Work out the finished part from the listing and answer in its coordinate system (mm). Face numbers are marked on the shaded views. A direction names the side the tool comes from. Round coordinates to 2 decimals unless told otherwise and drop trailing zeros. Loops run counter-clockwise (first coordinate to the right, second up) from the corner with the lowest first, then second, coordinate; pieces in that order, holes last.
from build123d import *

# Parameters (mm, degrees)
BOSS_EXTRUDE1_DEPTH = 30
SKETCH2_W           = 10
SKETCH2_H           = 20
SKETCH2_R           = 2.25
BOSS_EXTRUDE2_DEPTH = 4
SKETCH3_W           = 20
SKETCH3_H           = 10
CUT_EXTRUDE1_DEPTH  = 5
FILLET1_R           = 4
CHAMFER1_SIZE       = 14
CHAMFER1_SIZE2      = 16.684550296


with BuildPart() as part:
    # Sketch1 → Boss-Extrude1 (new body)
    with BuildSketch(Plane(origin=(0, 0, 0), x_dir=(0, 0, -1), z_dir=(1, 0, 0))):
        Polygon((0, 20), (20, 40), (20, 20), (20, 0), (0, 0), align=None)
    extrude(amount=BOSS_EXTRUDE1_DEPTH)

    # Sketch2 → Boss-Extrude2 (add)
    with BuildSketch(Plane.XY):
        with Locations((-5, 10)):
            Rectangle(SKETCH2_W, SKETCH2_H)
        with Locations((-5, 10)):
            Circle(SKETCH2_R, mode=Mode.SUBTRACT)
        with Locations((35, 10)):
            Rectangle(SKETCH2_W, SKETCH2_H)
        with Locations((35, 10)):
            Circle(SKETCH2_R, mode=Mode.SUBTRACT)
    extrude(amount=-BOSS_EXTRUDE2_DEPTH)

    # Sketch3 → Cut-Extrude1 (cut)
    with BuildSketch(Plane(origin=(0, 10, 10), x_dir=(1, 0, 0), z_dir=(0, 0.707106781, 0.707106781))):
        with Locations((15, 26.142135624)):
            Rectangle(SKETCH3_W, SKETCH3_H)
    extrude(amount=-CUT_EXTRUDE1_DEPTH, mode=Mode.SUBTRACT)

    # Fillet1
    fillet1_edges = [part.edges().sort_by_distance(p)[0] for p in [
        (15, 40, -20),
    ]]
    fillet(fillet1_edges, radius=FILLET1_R)

    # Chamfer1
    chamfer1_edges = [part.edges().sort_by_distance(p)[0] for p in [
        (15, 0, -20),
    ]]
    chamfer1_side = [part.faces().sort_by_distance(p)[0] for p in [
        (15, 0, -9.058823529),
    ]]
    chamfer(chamfer1_edges, length=CHAMFER1_SIZE, length2=CHAMFER1_SIZE2, reference=chamfer1_side[0])


solid = part.part
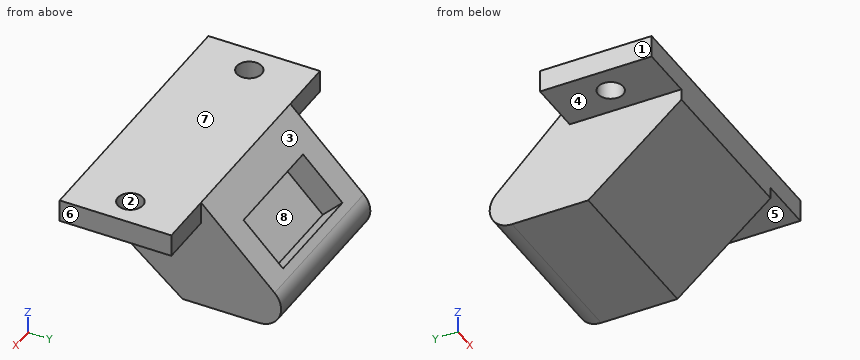
Item 1: Determine the mould class of the marked faces 1, 2 and 3 for opening direction X: pulls with the +X half, pulls with the -X half, needs draft (parallel to the pull), parting line crosses it, or undercut.
Item 2: Each of these flat-tipped pins is pushed along its axis until it touches: P1, Ø7, axis at x = -5, y = 10, coming from the +Z side; P2, Ø3, axis at y = 25.5, z = -8.5, coming from the +X side; P3, Ø10, axis at x = 7, y = 7, coming from the -Z side; P4, Ø6, axis at y = 12, z = -13.5, coming from the -X side. Where does it stop, or does it pass through?
Item 3: Section D-D, the plane y = 5.5 is taken. Give the vertices of the cut face in (x, z), plus the area to 3 significant figures.
Item 4: Section A-A, the plane x = 35 is taken. Give the vertices of the cut face in (y, z), plus the area to 3 significant figures.
Item 5: Section C-C, the plane x = 1.5 is taken. Give the vertices of the cut face in (y, z).
Item 6: Straight lines are drawn through the part: line 1 (Y direction, x = 35, z = -2.8); line 2 (X direction, y = 22.5, z = -8.5); line 3 (Z direction, x = 38, y = 9). For each, find the intervals that lie inside material, in ascending order.
Item 7: Section B-B, the plane y = 10 is taken. Give the vertices of the cut face in (x, z).
Item 8: For the marked faces 4, 5, 6, 7 and 8, determine the directions among +Z, -Z, +X, -X, +Y, -Y from which every point of the face is accessible in a straight line to the end or side of a thin tool.
Answer below:
1. face 1: pulls with the -X half
1. face 2: undercut
1. face 3: needs draft
2. P1: stops at z = 0
2. P2: stops at x = 30
2. P3: stops at z = -16.07
2. P4: stops at x = 0
3. outline: (-10, -4) - (0, -4) - (0, -10.62) - (30, -10.62) - (30, -4) - (40, -4) - (40, 0) - (-10, 0) - close
3. area: 398 mm2
4. outline: (0, -4) - (7.75, -4) - (7.75, 0) - (0, 0) - close; (12.25, -4) - (20, -4) - (20, 0) - (12.25, 0) - close
4. area: 62.0 mm2
5. outline: (0, -6) - (16.68, -20) - (30.34, -20) arc R4 ccw to (33.17, -13.17) - (20, 0) - (0, 0) - close
6. line 1: y = 0 to 7.75, 12.25 to 20
6. line 2: x = 0 to 5, 25 to 30
6. line 3: z = -4 to 0
7. outline: (-10, -4) - (-7.25, -4) - (-7.25, 0) - (-10, 0) - close; (-2.75, -4) - (0, -4) - (0, -14.39) - (30, -14.39) - (30, -4) - (32.75, -4) - (32.75, 0) - (-2.75, 0) - close; (37.25, -4) - (40, -4) - (40, 0) - (37.25, 0) - close
8. face 4: -Z, -X, +Y, -Y
8. face 5: -Z, +X, +Y, -Y
8. face 6: +Z, -Z, +X, +Y, -Y
8. face 7: +Z, +X, -X, +Y, -Y
8. face 8: none
